from build123d import *

# Parameters (mm, degrees)
SKETCH1_R           = 1.95
SKETCH1_R_2         = 4
SKETCH1_R_3         = 1.45
BOSS_EXTRUDE1_DEPTH = 5


with BuildPart() as part:
    # Sketch1 → Boss-Extrude1 (new body)
    with BuildSketch(Plane.XY.offset(-5.551615438)):
        with BuildLine():
            Line((-25.464626351, 10.13731735), (-12.396849296, 10.13731735))
            Line((-12.396849296, 10.13731735), (-12.396849296, 19.63731735))
            Line((-12.396849296, 19.63731735), (-7.414626351, 19.63731735))
            Line((-7.414626351, 19.63731735), (-7.414626351, 15.63731735))
            Line((-7.414626351, 15.63731735), (-8.864626351, 15.63731735))
            Line((-8.864626351, 15.63731735), (-8.864626351, 12.63731735))
            Line((-8.864626351, 12.63731735), (-7.414626351, 12.63731735))
            Line((-7.414626351, 12.63731735), (-7.414626351, 6.63731735))
            Line((-7.414626351, 6.63731735), (-3.514626351, 6.63731735))
            Line((-3.514626351, 6.63731735), (-3.514626351, 12.63731735))
            Line((-3.514626351, 12.63731735), (-2.064626351, 12.63731735))
            Line((-2.064626351, 12.63731735), (-2.064626351, 15.63731735))
            Line((-2.064626351, 15.63731735), (-3.514626351, 15.63731735))
            Line((-3.514626351, 15.63731735), (-3.514626351, 19.63731735))
            Line((-3.514626351, 19.63731735), (2.585373649, 19.63731735))
            Line((2.585373649, 19.63731735), (2.585373649, 15.63731735))
            Line((2.585373649, 15.63731735), (1.135373649, 15.63731735))
            Line((1.135373649, 15.63731735), (1.135373649, 12.63731735))
            Line((1.135373649, 12.63731735), (2.585373649, 12.63731735))
            Line((2.585373649, 12.63731735), (2.585373649, 6.63731735))
            Line((2.585373649, 6.63731735), (6.485373649, 6.63731735))
            Line((6.485373649, 6.63731735), (6.485373649, 12.63731735))
            Line((6.485373649, 12.63731735), (7.935373649, 12.63731735))
            Line((7.935373649, 12.63731735), (7.935373649, 15.63731735))
            Line((7.935373649, 15.63731735), (6.485373649, 15.63731735))
            Line((6.485373649, 15.63731735), (6.485373649, 19.63731735))
            Line((6.485373649, 19.63731735), (11.467596593, 19.63731735))
            Line((11.467596593, 19.63731735), (11.467596593, 10.13731735))
            Line((11.467596593, 10.13731735), (24.535373649, 10.13731735))
            ThreePointArc((24.535373649, 10.13731735), (25.949587211, 9.551530913), (26.535373649, 8.13731735))
            Line((26.535373649, 8.13731735), (26.535373649, -6.86268265))
            ThreePointArc((26.535373649, -6.86268265), (25.949587211, -8.276896212), (24.535373649, -8.86268265))
            Line((24.535373649, -8.86268265), (-10, -8.86268265))
            Line((-10, -8.86268265), (-25.464626351, -8.86268265))
            ThreePointArc((-25.464626351, -8.86268265), (-26.878839913, -8.276896212), (-27.464626351, -6.86268265))
            Line((-27.464626351, -6.86268265), (-27.464626351, 8.13731735))
            ThreePointArc((-27.464626351, 8.13731735), (-26.878839913, 9.551530913), (-25.464626351, 10.13731735))
        make_face()
        with Locations((-24.464626351, -4.36268265)):
            Circle(SKETCH1_R, mode=Mode.SUBTRACT)
        with Locations((23.535373649, -4.36268265)):
            Circle(SKETCH1_R, mode=Mode.SUBTRACT)
        with Locations((9.535373649, 0.63731735)):
            Circle(SKETCH1_R_2, mode=Mode.SUBTRACT)
        with Locations((-10.464626351, 0.63731735)):
            Circle(SKETCH1_R_3, mode=Mode.SUBTRACT)
        with Locations((-24.464626351, 2.63731735)):
            Circle(SKETCH1_R_3, mode=Mode.SUBTRACT)
        with Locations((23.535373649, 2.63731735)):
            Circle(SKETCH1_R_3, mode=Mode.SUBTRACT)
    extrude(amount=BOSS_EXTRUDE1_DEPTH)


solid = part.part
The listing builds one solid part. Answer for the finished solid, in the listing's coordinates (mm). A direction names the side the tool comes from. Give positions to 0.01 mm unless a question says otherwise; leave off trailing zeros. Loops run counter-clockwise (first coordinate to the right, second up) from the corner with the lowest first, then second, coordinate; pieces in that order, holes last. Notation, with made-up numbers: (67.25, -35.75) - (79.25, -35.75) arc R15 ccw to (79.25, -25.75) - close; hole circle Ø4 at (-13, 67). An arc over 180 degrees is marked (long way). Use one line per item in the form item = value.
1. Which of the six approach directions +Z, -Z, +X, -X, +Y, -Y give full straight-line access (tool end or side, diameter ignored) to faces 1 (the face through (11.468, 15, -3)), 2 (the face through (2.585, 10, -3)), 3 (the face through (-8, 15.637, -3))?
Calculated:
face_1 = +Z, -Z, +X, +Y
face_2 = +Z, -Z, +Y
face_3 = +Z, -Z
2. Section B-B on x = 23 is taken. Give the vertices of the cut face in (y, z), then the cut area to 3 significant figures.
Calculated:
outline = (-8.86, -5.55) - (-6.24, -5.55) - (-6.24, -0.55) - (-8.86, -0.55) - close; (-2.49, -5.55) - (1.29, -5.55) - (1.29, -0.55) - (-2.49, -0.55) - close; (3.98, -5.55) - (10.14, -5.55) - (10.14, -0.55) - (3.98, -0.55) - close
area = 62.8 mm^2
3. Section C-C on x = -20.5 is taken. Give the vertices of the cut face in (y, z), then the cut area to 3 significant figures.
Calculated:
outline = (-8.86, -5.55) - (10.14, -5.55) - (10.14, -0.55) - (-8.86, -0.55) - close
area = 95.0 mm^2
4. The mould has two halves that part along X. Classify faces 4 (the face through (-23.08, 3.07, -3.09)), 5 (the face through (-7.415, 18, -3)), 6 (the face through (25.965, -8.261, -3.087)), 7 (the face through (18, 10.137, -3)): pulls with the +X half, pulls with the -X half, needs draft (parallel to the pull), parting line crosses it, or undercut.
Calculated:
face_4 = undercut
face_5 = undercut
face_6 = pulls with the +X half
face_7 = needs draft
5. Find the intervals of material crossed by line 1 along X through (y, z) = (10.5, -2.05); line 2 along Y through (x, z) = (23.5, -3.8); line 3 along X through (y, z) = (7.5, -5.3), in increasing order. Write a range as [from, to].
Calculated:
line_1 = [-12.4, -7.41], [-3.51, 2.59], [6.49, 11.47]
line_2 = [-8.86, -6.31], [-2.41, 1.19], [4.09, 10.14]
line_3 = [-27.46, -7.41], [-3.51, 2.59], [6.49, 26.54]
6. Section A-A on y = 17.5 is taken. Give the vertices of the cut face in (x, z), then the cut area to 3 significant figures.
Calculated:
outline = (-12.4, -5.55) - (-7.41, -5.55) - (-7.41, -0.55) - (-12.4, -0.55) - close; (-3.51, -5.55) - (2.59, -5.55) - (2.59, -0.55) - (-3.51, -0.55) - close; (6.49, -5.55) - (11.47, -5.55) - (11.47, -0.55) - (6.49, -0.55) - close
area = 80.3 mm^2
7. Given pin 1 Ø1.5 at (y, z) = (10, -3.5) entering from -X; pin 2 Ø0.9 at (y, z) = (13.5, -3.5) entering from -X; pin 3 Ø1.5 at (y, z) = (9.5, -2) entering from -X, each flat-ended and moving along its own axis, determine where each tip first touches the part or whether it passes through.
Calculated:
pin_1 = -27.13
pin_2 = -12.4
pin_3 = -27.37
8. Section D-D on z = -2.65 is taken. Count the separate pieces of the cut face and the enclosed holes in it, then the cut area to 3 significant figures.
Calculated:
separate_pieces = 1
enclosed_holes = 6
area = 1,040 mm^2
